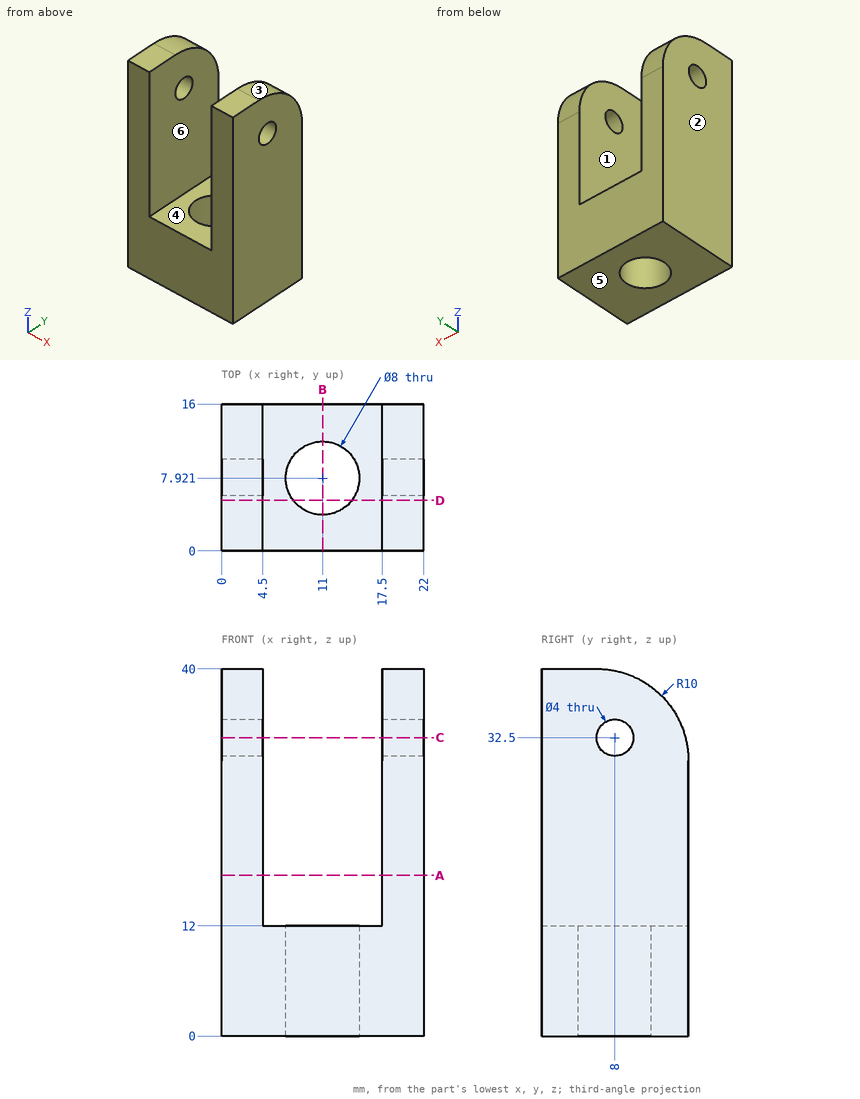
Study the drawing (mm; zero at the part's minimum x, y, z) and answer. A direction names the side the tool comes from. Give positions to 0.01 mm unless a question says otherwise; leave off trailing zeros. Write each loop counter-clockwise with the first axis right and the second up, starting at its lowest first coordinate (ties: lowest second). Pieces come first, ordered by that corner, then holes.
Item 1: Flat-ended cylindrical pins translate along their axes: P1, Ø1, axis at x = 18, y = 10, coming from the +Z side; P2, Ø6.5, axis at x = 9.5, y = 12, coming from the +Z side. Find the tip coordinate at first contact, or state that the pin passes through.
Item 2: Section A-A, the plane z = 17.5 is taken. Write down the section's boundary in (x, y).
Item 3: Section C-C, the plane z = 32.5 is taken. Write down the section's boundary in (x, y), plus the area to 3 significant figures.
Item 4: Which of the six approach directions +Z, -Z, +X, -X, +Y, -Y give full straight-line access (tool end or side, diameter ignored) to the marked faces 5 and 6?
Item 5: Section B-B, the plane x = 11 is taken. Write down the section's boundary in (y, z), plus the area to 3 significant figures.
Item 6: Find the intervals of material crossed by line 1 along Y through (x, z) = (11, 2.5); line 2 along X through (y, z) = (0.5, 22); line 3 along X through (y, z) = (6, 5.5), in increasing order.
Item 7: Section D-D, the plane y = 5.5 is taken. Write down the section's boundary in (x, z), plus the area to 3 significant figures.
Item 8: Determine the mould class of the marked faces 1, 2, 3 and 4 for opening direction X: released by +X, released by -X, zero draft, split by the parting line, or undercut.
Completed:
1. P1: stops at z = 39.37
1. P2: stops at z = 12
2. outline: (0, 0) - (4.5, 0) - (4.5, 16) - (0, 16) - close; (17.5, 0) - (22, 0) - (22, 16) - (17.5, 16) - close
3. outline: (0, 0) - (4.5, 0) - (4.5, 6) - (0, 6) - close; (0, 10) - (4.5, 10) - (4.5, 15.68) - (0, 15.68) - close; (17.5, 0) - (22, 0) - (22, 6) - (17.5, 6) - close; (17.5, 10) - (22, 10) - (22, 15.68) - (17.5, 15.68) - close
3. area: 105 mm2
4. face 5: -Z, +X, -X, +Y, -Y
4. face 6: +Z, +Y, -Y
5. outline: (0, 0) - (3.92, 0) - (3.92, 12) - (0, 12) - close; (11.92, 0) - (16, 0) - (16, 12) - (11.92, 12) - close
5. area: 96.0 mm2
6. line 1: y = 0 to 3.92, 11.92 to 16
6. line 2: x = 0 to 4.5, 17.5 to 22
6. line 3: x = 0 to 7.49, 14.51 to 22
7. outline: (0, 0) - (7.82, 0) - (7.82, 12) - (4.5, 12) - (4.5, 40) - (0, 40) - close; (14.18, 0) - (22, 0) - (22, 40) - (17.5, 40) - (17.5, 12) - (14.18, 12) - close
7. area: 440 mm2
8. face 1: undercut
8. face 2: released by -X
8. face 3: zero draft
8. face 4: undercut
